Part model, mm, in its own coordinate system. A direction names the side the tool comes from. Round coordinates to 2 decimals unless told otherwise and drop trailing zeros. Loops run counter-clockwise (first coordinate to the right, second up) from the corner with the lowest first, then second, coordinate; pieces in that order, holes last. Notation, with made-up numbers: (0, 68.25) - (42, 68.25) arc R30 cw to (42, 93.25) - close; hole circle Ø4 at (19, 12). An arc over 180 degrees is marked (long way). Put each result on its own line as item: value.
from build123d import *

# Parameters (mm, degrees)
SKETCH_1_R          = 22.5
SKETCH_1_R_2        = 2.15
EXTRUDE_1_DEPTH     = 10.4
SKETCH_3_R          = 4
SKETCH_3_R_2        = 2.15
CUT_EXTRUDE_1_DEPTH = 5
SKETCH_4_R          = 2.1
CUT_EXTRUDE_2_DEPTH = 34.476260245
SKETCH_6_R          = 22.5
CUT_EXTRUDE_3_DEPTH = 2


with BuildPart() as part:
    # 草图1 → 凸台-拉伸1 (new body)
    with BuildSketch(Plane(origin=(0, 0, 0), x_dir=(1, 0, 0), z_dir=(0, 1, 0))):
        with Locations(Location((0, 0, 0), (0, 0, 270))):
            Circle(SKETCH_1_R)
        with Locations(Location((0, 17.25, 0), (0, 0, 270))):
            Circle(SKETCH_1_R_2, mode=Mode.SUBTRACT)
        with Locations(Location((14.938938215, 8.625, 0), (0, 0, 270))):
            Circle(SKETCH_1_R_2, mode=Mode.SUBTRACT)
        with Locations(Location((14.938938215, -8.625, 0), (0, 0, 270))):
            Circle(SKETCH_1_R_2, mode=Mode.SUBTRACT)
        with Locations(Location((0, -17.25, 0), (0, 0, 270))):
            Circle(SKETCH_1_R_2, mode=Mode.SUBTRACT)
        with Locations(Location((-14.938938215, -8.625, 0), (0, 0, 270))):
            Circle(SKETCH_1_R_2, mode=Mode.SUBTRACT)
        with Locations(Location((-14.938938215, 8.625, 0), (0, 0, 270))):
            Circle(SKETCH_1_R_2, mode=Mode.SUBTRACT)
    extrude(amount=EXTRUDE_1_DEPTH)

    # 草图3 → 切除-拉伸1 (cut)
    # profile 1 of 6: a face of its own
    with BuildSketch(Plane.XZ):
        with Locations(Location((0, 17.25, 0), (0, 0, 270))):
            Circle(SKETCH_3_R)
        with Locations(Location((0, 17.25, 0), (0, 0, 270))):
            Circle(SKETCH_3_R_2, mode=Mode.SUBTRACT)
    # profile 2 of 6: a face of its own
    with BuildSketch(Plane.XZ):
        with Locations(Location((14.938938215, 8.625, 0), (0, 0, 270))):
            Circle(SKETCH_3_R)
        with Locations(Location((14.938938215, 8.625, 0), (0, 0, 270))):
            Circle(SKETCH_3_R_2, mode=Mode.SUBTRACT)
    # profile 3 of 6: a face of its own
    with BuildSketch(Plane.XZ):
        with Locations(Location((14.938938215, -8.625, 0), (0, 0, 270))):
            Circle(SKETCH_3_R)
        with Locations(Location((14.938938215, -8.625, 0), (0, 0, 270))):
            Circle(SKETCH_3_R_2, mode=Mode.SUBTRACT)
    # profile 4 of 6: a face of its own
    with BuildSketch(Plane.XZ):
        with Locations(Location((0, -17.25, 0), (0, 0, 270))):
            Circle(SKETCH_3_R)
        with Locations(Location((0, -17.25, 0), (0, 0, 270))):
            Circle(SKETCH_3_R_2, mode=Mode.SUBTRACT)
    # profile 5 of 6: a face of its own
    with BuildSketch(Plane.XZ):
        with Locations(Location((-14.938938215, -8.625, 0), (0, 0, 270))):
            Circle(SKETCH_3_R)
        with Locations(Location((-14.938938215, -8.625, 0), (0, 0, 270))):
            Circle(SKETCH_3_R_2, mode=Mode.SUBTRACT)
    # profile 6 of 6: a face of its own
    with BuildSketch(Plane.XZ):
        with Locations(Location((-14.938938215, 8.625, 0), (0, 0, 270))):
            Circle(SKETCH_3_R)
        with Locations(Location((-14.938938215, 8.625, 0), (0, 0, 270))):
            Circle(SKETCH_3_R_2, mode=Mode.SUBTRACT)
    extrude(amount=-CUT_EXTRUDE_1_DEPTH, mode=Mode.SUBTRACT)

    # 草图4 → 切除-拉伸2 (cut, through all)
    with BuildSketch(Plane.XZ):
        with BuildLine():
            ThreePointArc((5.05, 8.746856578), (2.181346652, 7.97820323), (2.95, 5.109549882))
            Line((2.95, 5.109549882), (5.05, 8.746856578))
        make_face()
        with BuildLine():
            Line((5.05, 8.746856578), (2.95, 5.109549882))
            ThreePointArc((2.95, 5.109549882), (5.05, 5.109549882), (6.1, 6.92820323))
            ThreePointArc((6.1, 6.92820323), (5.818653348, 7.97820323), (5.05, 8.746856578))
        make_face()
        with Locations(Location((8, 0, 0), (0, 0, 270))):
            Circle(SKETCH_4_R)
        with Locations(Location((-4, 6.92820323, 0), (0, 0, 270))):
            Circle(SKETCH_4_R)
        with Locations(Location((-8, 0, 0), (0, 0, 270))):
            Circle(SKETCH_4_R)
        with Locations(Location((-4, -6.92820323, 0), (0, 0, 270))):
            Circle(SKETCH_4_R)
        with Locations(Location((4, -6.92820323, 0), (0, 0, 270))):
            Circle(SKETCH_4_R)
    extrude(amount=-CUT_EXTRUDE_2_DEPTH, mode=Mode.SUBTRACT)

    # 草图6 → 切除-拉伸3 (cut)
    with BuildSketch(Plane.XZ):
        with Locations(Location((0, 0, 0), (0, 0, 270))):
            Circle(SKETCH_6_R)
    extrude(amount=-CUT_EXTRUDE_3_DEPTH, mode=Mode.SUBTRACT)


solid = part.part
1. Band-saw the part on B-B (z = 0). List the corners of the cut face in (x, y), plus the area to 3 significant figures.
A:
outline: (-22.5, 2) - (-10.1, 2) - (-10.1, 10.4) - (-22.5, 10.4) - close; (-5.9, 2) - (5.9, 2) - (5.9, 10.4) - (-5.9, 10.4) - close; (10.1, 2) - (22.5, 2) - (22.5, 10.4) - (10.1, 10.4) - close
area: 307 mm²
2. Band-saw the part on A-A (x = -7). List the corners of the cut face in (y, z), plus the area to 3 significant figures.
A:
outline: (2, -21.38) - (10.4, -21.38) - (10.4, -1.85) - (2, -1.85) - close; (2, 1.85) - (10.4, 1.85) - (10.4, 21.38) - (2, 21.38) - close
area: 328 mm²
3. Band-saw the part on C-C (y = 3.5). Give the number of separate pieces and of enclosed holes in the cut face, plus the area to 3 significant figures.
A:
separate pieces: 1
enclosed holes: 12
area: 1,210 mm²
4. Probe line 1 along X through (y, z) = (7.25, 0); line 2 along Z through (x, y) = (1.5, 3.5); line 3 along Z through (x, y) = (-14, 10). List the from-to ranges inside material, lowest first. Write a range as [from, to].
A:
line 1: x = [-22.5, -10.1], [-5.9, 5.9], [10.1, 22.5]
line 2: z = [-22.45, -20.96], [-13.54, 13.54], [20.96, 22.45]
line 3: z = [-17.61, -10.56], [-6.69, 6.69], [10.56, 17.61]
5. Pin check, flat tips, straight feed: P1, Ø7, axis at x = -14.94, z = -8.62, coming from the -Y side; P2, Ø5, axis at y = 4.5, z = 17.5, coming from the -X side; P3, Ø2, axis at y = 7.5, z = -17, coming from the -X side. Stop position of each tip, or through.
A:
P1: stops at y = 5
P2: stops at x = -16.77
P3: stops at x = -15.82
6. Band-saw the part on D-D (x = 0). List the corners of the cut face in (y, z).
A:
outline: (2, -22.5) - (10.4, -22.5) - (10.4, -19.4) - (5, -19.4) - (5, -21.25) - (2, -21.25) - close; (2, -13.25) - (5, -13.25) - (5, -15.1) - (10.4, -15.1) - (10.4, 15.1) - (5, 15.1) - (5, 13.25) - (2, 13.25) - close; (2, 21.25) - (5, 21.25) - (5, 19.4) - (10.4, 19.4) - (10.4, 22.5) - (2, 22.5) - close
7. Tool access for faces 1 (the cylindrical face through (12.505, 3.479, 11.799)), 2 (the cylindrical face through (-5.863, 6.141, 5.959)): list every direction of +Z, -Z, +X, -X, +Y, -Y with a clear straight run to the whole face (end or side of a thin tool).
A:
face 1: -Y
face 2: +Y, -Y
8. Two-plate mould, pull along Z, no slides. Class faces 3 (the flat face through (0, 10.4, 0)), 4 (the cylindrical face through (-5.918, 6.141, 0.273)), 5 (the cylindrical face through (-8.618, 6.141, 20.784)), 6 (the cylindrical face through (-2.434, 3.479, 20.424)): pulls with the +Z half, pulls with the -Z half, needs draft (parallel to the pull), parting line crosses it, or undercut.
A:
face 3: needs draft
face 4: undercut
face 5: parting line crosses it
face 6: undercut
